Work out the finished part from the listing and answer in its coordinate system (mm). Round coordinates to 2 decimals unless told otherwise and drop trailing zeros. Order: outer loops, then holes, each group sorted by start corner. A loop starts at its lowest first (then second) coordinate and runs counter-clockwise, first axis right, second up. Notation, with made-up numbers: M 70.25,77 L 76.25,77 A21 ccw 76.25,103 Z; hole C 17.25,58.25 d2. An arc over 180 degrees is marked long. Return JSON: item names as keys, results as strings.
from build123d import *

# Parameters (mm, degrees)
SKETCH_1_R      = 18
SKETCH_1_R_2    = 12
EXTRUDE_1_DEPTH = 28
FILLET_1_R      = 1


with BuildPart() as part:
    # Эскиз1 → Бобышка-Вытянуть1 (new, symmetric)
    with BuildSketch(Plane.XY):
        Circle(SKETCH_1_R)
        Circle(SKETCH_1_R_2, mode=Mode.SUBTRACT)
    extrude(amount=EXTRUDE_1_DEPTH, both=True)

    # Скругление1
    fillet_1_edges = [part.edges().sort_by_distance(p)[0] for p in [
        (-18, 0, -28),
        (-18, 0, 28),
        (-12, 0, -28),
        (-12, 0, 28),
    ]]
    fillet(fillet_1_edges, radius=FILLET_1_R)


solid = part.part
Item 1: The mould has two halves that part along X. Classify faces 1 (the cylindrical face through (-2.343, 17.847, 0.378)), 2 (the cylindrical face through (-11.99, 0.53, -0.38)), 3 (the flat face through (-4, -13, 28)): pulls with the +X half, pulls with the -X half, needs draft (parallel to the pull), parting line crosses it, or undercut.
Output:
{"face 1": "parting line crosses it", "face 2": "undercut", "face 3": "needs draft"}
Item 2: Consider line 1 along Y through (x, z) = (0, 9.5); line 2 along Y through (x, z) = (4, -22); line 3 along X through (y, z) = (10.5, -18.5). Determine where each line is inside the solid, lowest interval first. Write a range as [from, to].
Output:
{"line 1": "y = [-18, -12], [12, 18]", "line 2": "y = [-17.55, -11.31], [11.31, 17.55]", "line 3": "x = [-14.62, -5.81], [5.81, 14.62]"}
Item 3: Each of these flat-tipped pins is pushed along its axis until it touches: pin 1 (6 mm diameter, centred on x = 6, z = -12.5, fed in from +Y); pin 2 (2 mm diameter, centred on x = 12, z = -14, fed in from -Y); pin 3 (5 mm diameter, centred on y = 6.5, z = -21.5, fed in from +X). Where does it stop, or does it pass through?
Output:
{"pin 1": "stops at y = 17.75", "pin 2": "stops at y = -14.25", "pin 3": "stops at x = 17.55"}
Item 4: Find section C-C (z = -14). Determine the outline of the cut face in (x, y), plus the area to 3 significant figures.
Output:
{"outline": "C 0,0 d36; hole C 0,0 d24", "area": "565 mm^2"}
Item 5: Find section A-A (x = 0). Determine the outline of the cut face in (y, z).
Output:
{"outline": "M -18,-27 A1 ccw -17,-28 L -13,-28 A1 ccw -12,-27 L -12,27 A1 ccw -13,28 L -17,28 A1 ccw -18,27 Z; M 12,-27 A1 ccw 13,-28 L 17,-28 A1 ccw 18,-27 L 18,27 A1 ccw 17,28 L 13,28 A1 ccw 12,27 Z"}
